For this review, take the finished solid that the model builds, in its own axes (mm). A direction names the side the tool comes from. Coordinates: 2 decimals unless noted, no trailing zeros. Loops run counter-clockwise (first coordinate to the right, second up) from the corner with the lowest first, then second, coordinate; pieces in that order, holes last. Notation, with made-up numbers: (77, -24) -> (119, -24) arc R19 cw to (119, -14) -> close; hole circle Ø4 at (4, 23.5). An arc over 180 degrees is marked (long way). Answer in a Markdown table with one row per item.
from build123d import *

# Parameters (mm, degrees)
SKETCH1_R                 = 19.5
SKETCH1_R_2               = 18.5
EXTRUDE1_DEPTH            = 139.7
SKETCH4_R                 = 58.674
SKETCH4_R_2               = 19.5
EXTRUDE2_DEPTH            = 19.05
CUT_EXTRUDE1_REACH        = 164.485
SKETCH5_R                 = 4.2164
CIRPATTERN1_COUNT         = 10
F_4_40_TAPPED_HOLE2_D     = 2.2606
F_4_40_TAPPED_HOLE2_DEPTH = 7.62
F_4_40_TAPPED_HOLE2_TIP   = 0.679152758
SKETCH10_R                = 19
EXTRUDE3_DEPTH            = 25.4
EXTRUDE4_START            = 63.5
SKETCH12_R                = 21.5
SKETCH12_R_2              = 19
EXTRUDE4_DEPTH            = 63.5
FILLET1_R                 = 2.54
FILLET2_R                 = 2.54


with BuildPart() as part:
    # Sketch1 → Extrude1 (new body)
    with BuildSketch(Plane.XY):
        Circle(SKETCH1_R)
        Circle(SKETCH1_R_2, mode=Mode.SUBTRACT)
    extrude(amount=-EXTRUDE1_DEPTH)

    # Sketch4 → Extrude2 (add)
    with BuildSketch(Plane.XY):
        Circle(SKETCH4_R)
        Circle(SKETCH4_R_2, mode=Mode.SUBTRACT)
    extrude(amount=-EXTRUDE2_DEPTH)

    # Sketch5 → Cut-Extrude1 (cut, up to next)
    with BuildSketch(Plane.XY, mode=Mode.PRIVATE) as cut_extrude1_sk1:
        with Locations((0, 51.181)):
            Circle(SKETCH5_R)
    cut_extrude1_tool1 = extrude(cut_extrude1_sk1.sketch, amount=-CUT_EXTRUDE1_REACH, mode=Mode.PRIVATE) & part.part
    cut_extrude1 = cut_extrude1_tool1.solids().sort_by_distance((0, 51.181, 0))[0]
    add(cut_extrude1, mode=Mode.SUBTRACT)

    # CirPattern1: Cut-Extrude1 ×10 about axis
    cirpattern1_axis = Axis((0, 0, 0), (0, 0, 1))
    for i in range(1, CIRPATTERN1_COUNT):
        add(cut_extrude1.rotate(cirpattern1_axis, i * 360 / CIRPATTERN1_COUNT), mode=Mode.SUBTRACT)

    # #4-40 Tapped Hole2
    with Locations(Plane.XY):
        with Locations((15, -15), (-15, -15), (-15, 15), (15, 15), (0, 21.213203436), (-21.213203436, 0), (21.213203436, 0), (0, -21.213203436)):
            Hole(F_4_40_TAPPED_HOLE2_D / 2, depth=F_4_40_TAPPED_HOLE2_DEPTH)
            with Locations((0, 0, -(F_4_40_TAPPED_HOLE2_DEPTH + F_4_40_TAPPED_HOLE2_TIP / 2))):  # 118° drill point
                Cone(0, F_4_40_TAPPED_HOLE2_D / 2, F_4_40_TAPPED_HOLE2_TIP, mode=Mode.SUBTRACT)

    # Sketch10 → Extrude3 (cut)
    with BuildSketch(Plane(origin=(0, 0, -139.7), x_dir=(-1, 0, 0), z_dir=(0, 0, -1))):
        Circle(SKETCH10_R)
    extrude(amount=-EXTRUDE3_DEPTH, mode=Mode.SUBTRACT)

    # Sketch11 → Revolve1 (revolve)
    with BuildSketch(Plane(origin=(0, 0, 0), x_dir=(1, 0, 0), z_dir=(0, 1, 0)), mode=Mode.PRIVATE) as revolve1_sk:
        Polygon((-15, 139.7), (-15, 139.2), (-16.440598923, 139.2), (-18.75, 135.2), (-18.75, 130.320377846), (-19.25, 130.320377846), (-19.25, 135.333974596), (-16.729274058, 139.7), align=None)
    revolve(revolve1_sk.sketch.rotate(Axis((0, 0, -123.436944837), (0, 0, -1)), 180), axis=Axis((0, 0, -123.436944837), (0, 0, -1)))

    # Sketch12 → Extrude4 (add)
    with BuildSketch(Plane(origin=(0, 0, -19.05), x_dir=(-1, 0, 0), z_dir=(0, 0, -1)).offset(EXTRUDE4_START)):
        with Locations(Location((0, 0, 0), (0, 0, 180))):
            Circle(SKETCH12_R)
        Circle(SKETCH12_R_2, mode=Mode.SUBTRACT)
    extrude(amount=-EXTRUDE4_DEPTH)

    # Fillet1
    # the kernel refuses this fillet: 2.54 mm, written as the material it takes off along each edge
    with BuildSketch(Plane(origin=(0, 0, -82.55), x_dir=(1, 0, 0), z_dir=(0, 1, 0))) as fillet1_piece_1:
        with BuildLine():
            CenterArc((18.96, -2.481934729), FILLET1_R, 0, 77.725329785)
            Line((21.5, -2.481934729), (21.5508, -2.481934729))
            Line((21.5508, -2.481934729), (21.5508, 0))
            Line((21.5508, 0), (21.5, 0.0508))
            ThreePointArc((21.5, 0.0508), (20.5, 0.0508), (19.5108, 0.049638695))
            Line((19.5108, 0.049638695), (19.5, 0))
        make_face()
    revolve(axis=Axis((0, 0, -82.55), (0, 0, -1)), mode=Mode.SUBTRACT)

    # Fillet2
    fillet2_edges = [part.edges().sort_by_distance(p)[0] for p in [
        (-19.5, 0, -82.55),
    ]]
    fillet(fillet2_edges, radius=FILLET2_R)


solid = part.part
Item 1: For faces 1 (the cylindrical face through (-4.01, -18.06, -56.35)), 2 (the cylindrical face through (8.652, 16.634, -132.726)), 3 (the cylindrical face through (-2.799, -21.317, -49.986)), list the 3-axis set-ups (+Z, -Z, +X, -X, +Y, -Y) from which the entire face can be reached by the end or side of a thin tool; tool diameter is ignored.
Worked answers:
| item | result |
|---|---|
| face 1 | +Z |
| face 2 | none |
| face 3 | -Z |
Item 2: Take a section at B-B, the plane z = -54. State the section outline as (x, y) points.
Worked answers:
| item | result |
|---|---|
| outline | circle Ø43 at (0, 0); hole circle Ø37 at (0, 0) |
Item 3: Take a section at A-A, the plane y = 42. State the section outline as (x, z) points, and give its area (3 significant figures).
Worked answers:
| item | result |
|---|---|
| outline | (-40.97, -19.05) -> (-34.26, -19.05) -> (-34.26, 0) -> (-40.97, 0) -> close; (-25.91, -19.05) -> (25.91, -19.05) -> (25.91, 0) -> (-25.91, 0) -> close; (34.26, -19.05) -> (40.97, -19.05) -> (40.97, 0) -> (34.26, 0) -> close |
| area | 1,240 mm² |
Item 4: Insertion check: pin 1 (4 mm diameter, centred on x = -32, y = 39.5, fed in from -Z); pin 2 (23 mm diameter, centred on x = 0, y = 0, fed in from +Z); pin 3 (10 mm diameter, centred on x = 4.5, z = -17, fed in from -Y); pin 4 (1.8 mm diameter, centred on x = 15, y = -15, fed in from +Z). Each pin has a flat end and moves straight along its axis. Give the tip position at first contact, or say it passes through.
Worked answers:
| item | result |
|---|---|
| pin 1 | z = -19.05 |
| pin 2 | through |
| pin 3 | y = -58.67 |
| pin 4 | z = -7.76 |
Item 5: Take a section at C-C, the plane x = 37.5. State the section outline as (y, z) points.
Worked answers:
| item | result |
|---|---|
| outline | (-45.13, -19.05) -> (45.13, -19.05) -> (45.13, 0) -> (-45.13, 0) -> close |
Item 6: For L1, parallel to Y at x = 0, z = -2; L2, parallel to X at y = 15, z = -1.5; L3, parallel to X at y = 1, z = -42, list the stretches that pass through material, from the lowest coordinate up.
Worked answers:
| item | result |
|---|---|
| L1 | -58.67 to -55.4, -46.96 to -22.34, -20.08 to -18.5, 18.5 to 20.08, 22.34 to 46.96, 55.4 to 58.67 |
| L2 | -56.72 to -52.81, -44.54 to -16.13, -13.87 to -10.83, 10.83 to 13.87, 16.13 to 44.54, 52.81 to 56.72 |
| L3 | -21.48 to -18.47, 18.47 to 21.48 |
Item 7: The part is to be moulded in two halves that separate along X. For faces 4 (the cylindrical face through (18.6, 5.86, -111.51)), 5 (the cylindrical face through (8.06, -12.65, -139.45)), 6 (the flat face through (18.7, -4.2, -139.7)), say which applies: +X half, -X half, draft (parallel to the pull), parting line (faces both ways), or undercut.
Worked answers:
| item | result |
|---|---|
| face 4 | parting line |
| face 5 | undercut |
| face 6 | draft |
